Part print with two shaded views. Sizes in mm from the minimum x, y, z corner. Coordinates: 2 decimals unless noted, no trailing zeros. Order: outer loops, then holes, each group sorted by start corner. A loop starts at its lowest first (then second) coordinate and runs counter-clockwise, first axis right, second up.
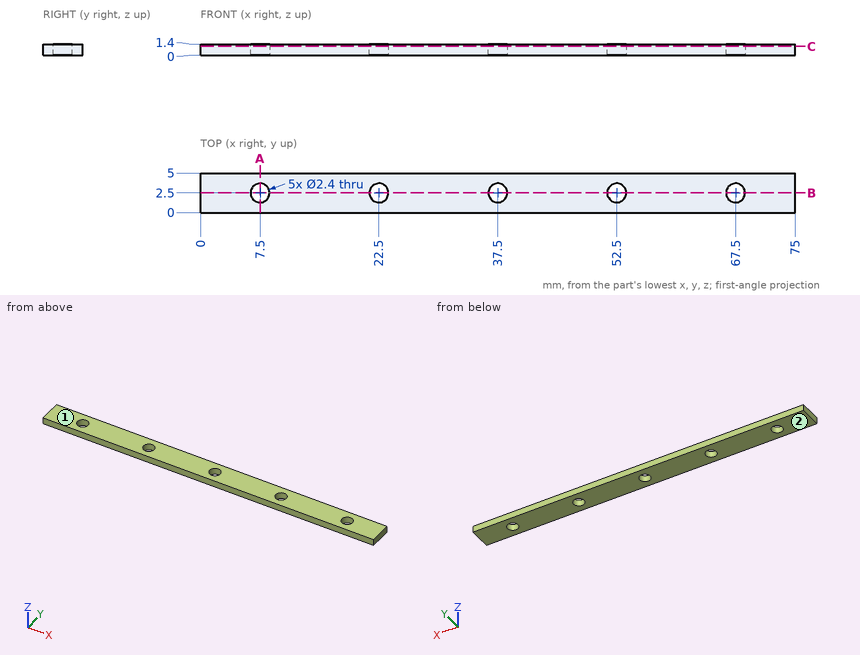
Q1. Cut at B-B on y = 2.5. Write the cut outline in (x, z).
Results list:
outline: (0, 0) - (6.3, 0) - (6.3, 1.4) - (0, 1.4) - close; (8.7, 0) - (21.3, 0) - (21.3, 1.4) - (8.7, 1.4) - close; (23.7, 0) - (36.3, 0) - (36.3, 1.4) - (23.7, 1.4) - close; (38.7, 0) - (51.3, 0) - (51.3, 1.4) - (38.7, 1.4) - close; (53.7, 0) - (66.3, 0) - (66.3, 1.4) - (53.7, 1.4) - close; (68.7, 0) - (75, 0) - (75, 1.4) - (68.7, 1.4) - close
Q2. Cut at A-A on x = 7.5. Write the cut outline in (y, z).
Results list:
outline: (0, 0) - (1.3, 0) - (1.3, 1.4) - (0, 1.4) - close; (3.7, 0) - (5, 0) - (5, 1.4) - (3.7, 1.4) - close
Q3. Wall check: line 1 along Y through (x, z) = (52.5, 1.05); line 2 along X through (y, z) = (2.8, 0.15); line 3 along X through (y, z) = (2.9, 0.25). Give the ranges that are in metal, low to high.
Results list:
line 1: y = 0 to 1.3, 3.7 to 5
line 2: x = 0 to 6.34, 8.66 to 21.34, 23.66 to 36.34, 38.66 to 51.34, 53.66 to 66.34, 68.66 to 75
line 3: x = 0 to 6.37, 8.63 to 21.37, 23.63 to 36.37, 38.63 to 51.37, 53.63 to 66.37, 68.63 to 75
Q4. Pin check, flat tip, straight feed: pin 1 Ø2 at (x, y) = (22.5, 2.5) entering from -Z. Stop position of the tip, or through.
Results list:
pin 1: passes through
Q5. Mould opens along Z. For the marked faces 1 and 2 say: pulls with the +Z half, pulls with the -Z half, needs draft (parallel to the pull), parting line crosses it, or undercut.
Results list:
face 1: pulls with the +Z half
face 2: pulls with the -Z half
Q6. Cut at C-C on z = 1.1. Write the cut outline in (x, y), and give its area (3 significant figures).
Results list:
outline: (0, 0) - (75, 0) - (75, 5) - (0, 5) - close; hole circle Ø2.4 at (7.5, 2.5); hole circle Ø2.4 at (22.5, 2.5); hole circle Ø2.4 at (37.5, 2.5); hole circle Ø2.4 at (52.5, 2.5); hole circle Ø2.4 at (67.5, 2.5)
area: 352 mm2
